Could you check a few things on this model? Use its own coordinates, in mm. A direction names the side the tool comes from. Coordinates: 2 decimals unless noted, no trailing zeros. Loops run counter-clockwise (first coordinate to the right, second up) from the corner with the lowest first, then second, coordinate; pieces in that order, holes last.
1) Imagine slicing it at C-C on x = 6.5. Please give me the cut outline in (y, z).
2) If I drill on line 1 along Z through (x, y) = (9.25, -1.5); line 2 along Z through (x, y) = (9, 12.5); line 3 along Y through (x, z) = (5.5, 10.5), over which ranges is the centre line in solid material (lowest first)?
3) Imagine slicing it at A-A on z = 0. Please give me the cut outline in (x, y).
4) Thinking about a two-plate mould opening in Y: for faces 3 (the face through (4.935, -15.252, -48.433)), 4 (the face through (5, 5, -17.5)), 5 (the face through (9.734, -1, 22)), which applies, released by +Y, released by -Y, zero draft, split by the parting line, or undercut?
5) Imagine slicing it at D-D on y = -33. Please give me the cut outline in (x, z).
6) Will these pins go through, and if not, where does the flat tip stop? P1, Ø3, axis at x = 4.5, z = 16.5, coming from the -Y side; P2, Ø3, axis at x = 5, z = 8, coming from the +Y side; P3, Ø1.5, axis at x = 8, y = -6, coming from the -Z side; P4, Ø4, axis at y = 27.5, z = -12, coming from the -X side.
7) For faces 1 (the face through (0, -1, 22)), 2 (the face through (4.8, -14.65, -14.49)), which set-ups out of +Z, -Z, +X, -X, +Y, -Y let a thin tool reach every point of the face, with its end or its side?
```python
from build123d import *

# Parameters (mm, degrees)
ESQUISSE1_W             = 9.734075662
ESQUISSE1_H             = 50.777874564
ESQUISSE2_W             = 35
ESQUISSE2_H             = 35
ENL_V_MAT_EXTRU_1_DEPTH = 10.734075662
CONG_2_R                = 10


with BuildPart() as part:
    # Esquisse1 → Révolution1 (revolve)
    with BuildSketch(Plane.XY, mode=Mode.PRIVATE) as r_volution1_sk:
        with Locations((4.867037831, 25.388937282)):
            Rectangle(ESQUISSE1_W, ESQUISSE1_H)
    revolve(r_volution1_sk.sketch.rotate(Axis((9.734075662, 0, 0), (-1, 0, 0)), 90), axis=Axis((9.734075662, 0, 0), (-1, 0, 0)))  # turned: the seam where the file's is

    # Esquisse2 → Enlèv. mat.-Extru.1 (cut, through all)
    with BuildSketch(Plane(origin=(9.734075662, 0, 0), x_dir=(0, 0, -1), z_dir=(1, 0, 0))):
        Rectangle(ESQUISSE2_W, ESQUISSE2_H)
    extrude(amount=-ENL_V_MAT_EXTRU_1_DEPTH, mode=Mode.SUBTRACT)

    # Congé2
    cong_2_edges = [part.edges().sort_by_distance(p)[0] for p in [
        (4.867037831, -17.5, -17.5),
    ]]
    fillet(cong_2_edges, radius=CONG_2_R)


solid = part.part
```
Filled in:
1. outline: circle Ø101.56 at (0, 0); hole (-17.5, -7.5) arc R10 ccw to (-7.5, -17.5) - (17.5, -17.5) - (17.5, 17.5) - (-17.5, 17.5) - close
2. line 1: z = -50.76 to -17.5, 17.5 to 50.76
2. line 2: z = -49.22 to -17.5, 17.5 to 49.22
2. line 3: y = -49.68 to -17.5, 17.5 to 49.68
3. outline: (0, -50.78) - (9.73, -50.78) - (9.73, -17.5) - (0, -17.5) - close; (0, 17.5) - (9.73, 17.5) - (9.73, 50.78) - (0, 50.78) - close
4. face 3: split by the parting line
4. face 4: undercut
4. face 5: zero draft
5. outline: (0, -38.59) - (9.73, -38.59) - (9.73, 38.59) - (0, 38.59) - close
6. P1: stops at y = -48.51
6. P2: stops at y = 50.36
6. P3: stops at z = -50.51
6. P4: stops at x = 0
7. face 1: +Z, -Z, -X, +Y, -Y
7. face 2: +X, -X
